```python
from build123d import *

# Parameters (mm, degrees)
F1_DEPTH  = 160
F3_DEPTH  = 160
F4_W      = 56.4157663456
F4_H      = 160
F5_DEPTH  = 4
F7_DEPTH  = 160
F10_DEPTH = 70
F11_R     = 2.25
F12_DEPTH = 4
F13_R     = 2.25
F14_DEPTH = 5


with BuildPart() as f1:
    # F0 (on Top) → F1 (new body)
    with BuildSketch(Plane.XY):
        with BuildLine():
            Line((-48.2078831728, -76), (48.2078831728, -76))
            ThreePointArc((48.2078831728, -76), (0, 90), (-48.2078831728, -76))
        make_face()
    extrude(amount=F1_DEPTH)

    # F2 (on face) → F3 (cut, through all)
    with BuildSketch(Plane.XY.offset(160)):
        with BuildLine():
            Line((-47.0319040652, -72), (47.0319040652, -72))
            ThreePointArc((47.0319040652, -72), (0, 86), (-47.0319040652, -72))
        make_face()
    extrude(amount=-F3_DEPTH, mode=Mode.SUBTRACT)

    # F4 (on face) → F5 (cut, through all)
    with BuildSketch(Plane.XZ.offset(76)):
        with Locations((0, 80)):
            Rectangle(F4_W, F4_H)
    extrude(amount=-F5_DEPTH, mode=Mode.SUBTRACT)

    # F6 (on Top) → F7 (join)
    with BuildSketch(Plane.XY):
        with BuildLine():
            ThreePointArc((43.9545219517, -62), (0, 76), (-43.9545219517, -62))
            Line((-43.9545219517, -62), (-28.2078831728, -62))
            Line((-28.2078831728, -62), (-28.2078831728, -59))
            Line((-28.2078831728, -59), (-42.9883705204, -59))
            ThreePointArc((-42.9883705204, -59), (0, 73), (42.9883705204, -59))
            Line((42.9883705204, -59), (28.2078831728, -59))
            Line((28.2078831728, -59), (28.2078831728, -62))
            Line((28.2078831728, -62), (43.9545219517, -62))
        make_face()
        Polygon((-28.2078831728, -62), (-43.9545219517, -62), (-46.9199158251, -72.0180869102), (-28.2078831728, -72.0180869102), align=None)
        Polygon((46.9199158251, -72.0180869102), (43.9545219517, -62), (28.2078831728, -62), (28.2078831728, -72.0180869102), align=None)
    extrude(amount=F7_DEPTH)


with BuildPart() as f1_1:
    # F8: moved
    add(f1.part.moved(Location((0, 0, -80))))

    # F9 (on Top) → F10 (cut, symmetric)
    with BuildSketch(Plane.XY):
        with BuildLine():
            Line((62.496284582, -59.0780366418), (67.8954018071, -59.0780366418))
            ThreePointArc((67.8954018071, -59.0780366418), (0.0239748666, 89.9999968067), (-67.9268674599, -59.0418552984))
            Line((-67.9268674599, -59.0418552984), (-62.5304671574, -59.0418552984))
            ThreePointArc((-62.5304671574, -59.0418552984), (0.0248874369, 85.9999963989), (62.496284582, -59.0780366418))
        make_face()
    extrude(amount=F10_DEPTH, both=True, mode=Mode.SUBTRACT)

    # F11 (on face) → F12 (join)
    with BuildSketch(Plane.XY.offset(80)):
        with BuildLine():
            ThreePointArc((-75.7423312883, 6.2529393893), (-80.5249171029, 8.4438861518), (-85.6809815951, 7.4006346283))
            ThreePointArc((-85.6809815951, 7.4006346283), (-86, 0), (-85.6809815951, -7.4006346283))
            ThreePointArc((-85.6809815951, -7.4006346283), (-80.5249171029, -8.4438861518), (-75.7423312883, -6.2529393893))
            ThreePointArc((-75.7423312883, -6.2529393893), (-76, 0), (-75.7423312883, 6.2529393893))
        make_face()
        with Locations((-81.5, 0)):
            Circle(F11_R, mode=Mode.SUBTRACT)
        with BuildLine():
            ThreePointArc((6.2529393893, 75.7423312883), (7.9183326783, 78.409691343), (8.5, 81.5))
            ThreePointArc((8.5, 81.5), (8.2205655019, 83.6615510241), (7.4006346283, 85.6809815951))
            ThreePointArc((7.4006346283, 85.6809815951), (0, 86), (-7.4006346283, 85.6809815951))
            ThreePointArc((-7.4006346283, 85.6809815951), (-8.4438861518, 80.5249171029), (-6.2529393893, 75.7423312883))
            ThreePointArc((-6.2529393893, 75.7423312883), (0, 76), (6.2529393893, 75.7423312883))
        make_face()
        with Locations((0, 81.5)):
            Circle(F11_R, mode=Mode.SUBTRACT)
        with BuildLine():
            ThreePointArc((85.6809815951, -7.4006346283), (86, 0), (85.6809815951, 7.4006346283))
            ThreePointArc((85.6809815951, 7.4006346283), (80.5249171029, 8.4438861518), (75.7423312883, 6.2529393893))
            ThreePointArc((75.7423312883, 6.2529393893), (76, 0), (75.7423312883, -6.2529393893))
            ThreePointArc((75.7423312883, -6.2529393893), (80.5249171029, -8.4438861518), (85.6809815951, -7.4006346283))
        make_face()
        with Locations((81.5, 0)):
            Circle(F11_R, mode=Mode.SUBTRACT)
        with BuildLine():
            ThreePointArc((90, 0), (88.8412649986, 4.2843702245), (85.6809815951, 7.4006346283))
            ThreePointArc((85.6809815951, 7.4006346283), (86, 0), (85.6809815951, -7.4006346283))
            ThreePointArc((85.6809815951, -7.4006346283), (88.8412649986, -4.2843702245), (90, 0))
        make_face()
        with BuildLine():
            ThreePointArc((-7.4006346283, 85.6809815951), (0, 86), (7.4006346283, 85.6809815951))
            ThreePointArc((7.4006346283, 85.6809815951), (4.2843702226, 88.8412649997), (-4.4e-09, 90))
            ThreePointArc((-4.4e-09, 90), (-4.2843702264, 88.8412649975), (-7.4006346283, 85.6809815951))
        make_face()
        with BuildLine():
            ThreePointArc((-85.6809815951, 7.4006346283), (-88.8412649971, 4.284370227), (-90, 5.8e-09))
            ThreePointArc((-90, 5.8e-09), (-88.841265, -4.284370222), (-85.6809815951, -7.4006346283))
            ThreePointArc((-85.6809815951, -7.4006346283), (-86, 0), (-85.6809815951, 7.4006346283))
        make_face()
    extrude(amount=-F12_DEPTH)

    # F13 (on face) → F14 (join)
    with BuildSketch(Plane(origin=(0, 0, -80), x_dir=(1, 0, 0), z_dir=(0, 0, -1))):
        with BuildLine():
            ThreePointArc((-75.7423312883, -6.2529393893), (-76, 0), (-75.7423312883, 6.2529393893))
            ThreePointArc((-75.7423312883, 6.2529393893), (-80.5249171029, 8.4438861518), (-85.6809815951, 7.4006346283))
            ThreePointArc((-85.6809815951, 7.4006346283), (-86, 0), (-85.6809815951, -7.4006346283))
            ThreePointArc((-85.6809815951, -7.4006346283), (-80.5249171029, -8.4438861518), (-75.7423312883, -6.2529393893))
        make_face()
        with Locations((-81.5, 0)):
            Circle(F13_R, mode=Mode.SUBTRACT)
        with BuildLine():
            ThreePointArc((-85.6809815951, -7.4006346283), (-86, 0), (-85.6809815951, 7.4006346283))
            ThreePointArc((-85.6809815951, 7.4006346283), (-88.8412649692, 4.2843702749), (-90, 1.165e-07))
            ThreePointArc((-90, 1.165e-07), (-88.8412650279, -4.2843701742), (-85.6809815951, -7.4006346283))
        make_face()
        with BuildLine():
            ThreePointArc((85.6809815951, 7.4006346283), (86, 0), (85.6809815951, -7.4006346283))
            ThreePointArc((85.6809815951, -7.4006346283), (88.8412649986, -4.2843702245), (90, 0))
            ThreePointArc((90, 0), (88.8412649986, 4.2843702245), (85.6809815951, 7.4006346283))
        make_face()
        with BuildLine():
            ThreePointArc((75.7423312883, 6.2529393893), (76, 0), (75.7423312883, -6.2529393893))
            ThreePointArc((75.7423312883, -6.2529393893), (80.5249171029, -8.4438861518), (85.6809815951, -7.4006346283))
            ThreePointArc((85.6809815951, -7.4006346283), (86, 0), (85.6809815951, 7.4006346283))
            ThreePointArc((85.6809815951, 7.4006346283), (80.5249171029, 8.4438861518), (75.7423312883, 6.2529393893))
        make_face()
        with Locations((81.5, 0)):
            Circle(F13_R, mode=Mode.SUBTRACT)
        with BuildLine():
            ThreePointArc((6.2529393893, -75.7423312883), (0, -76), (-6.2529393893, -75.7423312883))
            ThreePointArc((-6.2529393893, -75.7423312883), (-8.4438861518, -80.5249171029), (-7.4006346283, -85.6809815951))
            ThreePointArc((-7.4006346283, -85.6809815951), (0, -86), (7.4006346283, -85.6809815951))
            ThreePointArc((7.4006346283, -85.6809815951), (8.2205655019, -83.6615510241), (8.5, -81.5))
            ThreePointArc((8.5, -81.5), (7.9183326783, -78.409691343), (6.2529393893, -75.7423312883))
        make_face()
        with Locations((0, -81.5)):
            Circle(F13_R, mode=Mode.SUBTRACT)
        with BuildLine():
            ThreePointArc((7.4006346283, -85.6809815951), (0, -86), (-7.4006346283, -85.6809815951))
            ThreePointArc((-7.4006346283, -85.6809815951), (-4.2843702239, -88.8412649989), (1.4e-09, -90))
            ThreePointArc((1.4e-09, -90), (4.2843702252, -88.8412649982), (7.4006346283, -85.6809815951))
        make_face()
    extrude(amount=-F14_DEPTH)


solid = f1_1.part
```
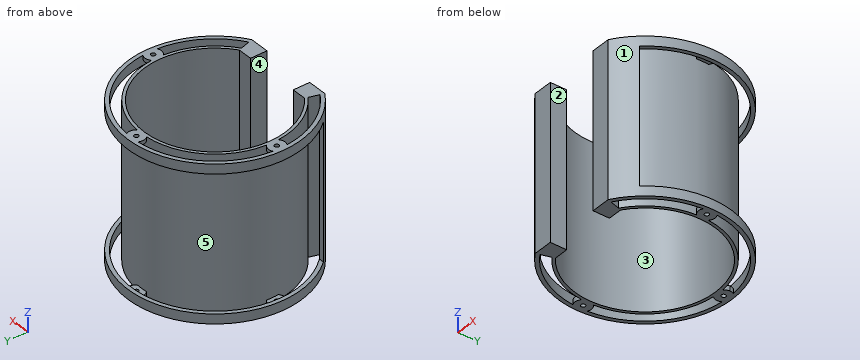
Geometry check sheet. Reference: the model listing, model coordinates, mm. Face numbers are marked on the shaded views. A direction names the side the tool comes from. Coordinates: 2 decimals unless noted, no trailing zeros. Loops run counter-clockwise (first coordinate to the right, second up) from the corner with the lowest first, then second, coordinate; pieces in that order, holes last.
Item 1: Sectioned sample at C-C, the plane y = 51. Record the boundary of the cut face in (x, z).
Item 2: Go/stop test with flat-tipped pins: pin 1 Ø1 at (y, z) = (14, 34) entering from -X; pin 2 Ø1.5 at (y, z) = (-27.5, -38) entering from -X; pin 3 Ø8 at (x, z) = (-17, -6.5) entering from +Y. Record where each tip stops, or that it passes through.
Item 3: Thickness scan on line 1 (Y direction, x = 0, z = 78); line 2 (Y direction, x = 47.5, z = -11); line 3 (X direction, y = -54, z = 42). Record the ranges inside material, lowest first.
Item 4: Sectioned sample at B-B, the plane z = -19. Record the boundary of the cut face in (x, y).
Item 5: Release check for a two-part mould opening along X. For the marked faces 1 and 2 record: released by +X, released by -X, zero draft, split by the parting line, or undercut.
Item 6: Sectioned sample at A-A, the plane y = -28.5. Record the boundary of the cut face in (x, z), then the cut area to 3 significant figures.
Item 7: Access from +Z, -Z, +X, -X, +Y, -Y to the whole of each face (thin tool, end or side, straight path). Record for the marked faces 3, 4 and 5.
Check result:
1. outline: (-74.16, -80) - (-69.25, -80) - (-69.25, -70) - (-74.16, -70) - close; (-74.16, 70) - (-69.25, 70) - (-69.25, 80) - (-74.16, 80) - close; (-56.35, -80) - (-52.23, -80) - (-52.23, 80) - (-56.35, 80) - close; (52.23, -80) - (56.35, -80) - (56.35, 80) - (52.23, 80) - close; (69.25, -80) - (74.16, -80) - (74.16, -70) - (69.25, -70) - close; (69.25, 70) - (74.16, 70) - (74.16, 80) - (69.25, 80) - close
2. pin 1: stops at x = -74.79
2. pin 2: stops at x = -71.14
2. pin 3: stops at y = 74.88
3. line 1: y = 73 to 79.25, 83.75 to 90
3. line 2: y = -76 to -71.69, -59.33 to -55.43, 55.43 to 59.33
3. line 3: x = -53.48 to -49.12, 49.12 to 53.48
4. outline: (-67.93, -59.04) arc R90 ccw to (-48.21, -76) - (-28.21, -76) - (-28.21, -59) - (-42.99, -59) arc R73 cw (long way) to (42.99, -59) - (28.21, -59) - (28.21, -76) - (48.21, -76) arc R90 ccw to (67.9, -59.08) - (62.5, -59.08) arc R86 cw to (47.03, -72) - (46.91, -72) - (43.95, -62) arc R76 ccw (long way) to (-43.95, -62) - (-46.91, -72) - (-47.03, -72) arc R86 cw to (-62.53, -59.04) - close
5. face 1: split by the parting line
5. face 2: undercut
6. outline: (-85.37, -80) - (-81.14, -80) - (-81.14, -70) - (-85.37, -70) - close; (-85.37, 70) - (-81.14, 70) - (-81.14, 80) - (-85.37, 80) - close; (-70.45, -80) - (-67.21, -80) - (-67.21, 80) - (-70.45, 80) - close; (67.21, -80) - (70.45, -80) - (70.45, 80) - (67.21, 80) - close; (81.14, -80) - (85.37, -80) - (85.37, -70) - (81.14, -70) - close; (81.14, 70) - (85.37, 70) - (85.37, 80) - (81.14, 80) - close
6. area: 1,210 mm2
7. face 3: +Z, -Z
7. face 4: +Z, -Z, -Y
7. face 5: none
